For this review, take the finished solid that the model builds, in its own axes (mm). A direction names the side the tool comes from. Give positions to 0.01 mm unless a question says otherwise; leave off trailing zeros. Order: outer loops, then holes, each group sorted by start corner. A loop starts at its lowest first (then second) coordinate and runs counter-clockwise, first axis right, second up.
from build123d import *

# Parameters (mm, degrees)
SKETCH_1_W                   = 200
SKETCH_1_H                   = 80
EXTRUDE_1_DEPTH              = 10
SKETCH_3_R                   = 9
CUT_EXTRUDE_1_DEPTH          = 5
HOLE_WIZARD_M2_1_D           = 2.4
HOLE_WIZARD_M2_1_CBORE_D     = 5
HOLE_WIZARD_M2_1_CBORE_DEPTH = 7.7
SKETCH_13_R                  = 1.7
CUT_EXTRUDE_3_DEPTH          = 109.166538264
SKETCH_14_R                  = 3.25
CUT_EXTRUDE_4_DEPTH          = 109.166538264
FILLET1_R                    = 10
SKETCH3_W                    = 12
SKETCH3_H                    = 12
CUT_EXTRUDE2_DEPTH           = 109.166538264


with BuildPart() as part:
    # 草图1 → 凸台-拉伸1 (new body)
    with BuildSketch(Plane(origin=(0, 0, 0), x_dir=(1, 0, 0), z_dir=(0, 1, 0))):
        Rectangle(SKETCH_1_W, SKETCH_1_H)
    extrude(amount=EXTRUDE_1_DEPTH)

    # 草图3 → 切除-拉伸1 (cut)
    with BuildSketch(Plane(origin=(0, 10, 0), x_dir=(1, 0, 0), z_dir=(0, 1, 0))):
        with Locations(Location((-70, 0, 0), (0, 0, 270))):
            Circle(SKETCH_3_R)
    extrude(amount=-CUT_EXTRUDE_1_DEPTH, mode=Mode.SUBTRACT)

    # M2 六角凹头螺钉的柱形沉头孔1 (through all)
    with Locations(Plane(origin=(0, 0, 0), x_dir=(-1, 0, 0), z_dir=(0, -1, 0))):
        with Locations((47.5, 8), (77.5, 8), (77.5, -8), (47.5, -8)):
            CounterBoreHole(HOLE_WIZARD_M2_1_D / 2, HOLE_WIZARD_M2_1_CBORE_D / 2, HOLE_WIZARD_M2_1_CBORE_DEPTH)

    # 草图13 → 切除-拉伸3 (cut, through all)
    with BuildSketch(Plane(origin=(0, 10, 0), x_dir=(1, 0, 0), z_dir=(0, 1, 0))):
        with Locations(Location((-20, 31.5, 0), (0, 0, 270))):
            Circle(SKETCH_13_R)
        with Locations(Location((4, 31.5, 0), (0, 0, 270))):
            Circle(SKETCH_13_R)
        with Locations(Location((28, 31.5, 0), (0, 0, 270))):
            Circle(SKETCH_13_R)
        with Locations(Location((52, 31.5, 0), (0, 0, 270))):
            Circle(SKETCH_13_R)
        with Locations(Location((76, 31.5, 0), (0, 0, 270))):
            Circle(SKETCH_13_R)
        with Locations(Location((4, 10.5, 0), (0, 0, 270))):
            Circle(SKETCH_13_R)
        with Locations(Location((28, 10.5, 0), (0, 0, 270))):
            Circle(SKETCH_13_R)
        with Locations(Location((52, 10.5, 0), (0, 0, 270))):
            Circle(SKETCH_13_R)
        with Locations(Location((76, 10.5, 0), (0, 0, 270))):
            Circle(SKETCH_13_R)
        with Locations(Location((4, -10.5, 0), (0, 0, 270))):
            Circle(SKETCH_13_R)
        with Locations(Location((28, -10.5, 0), (0, 0, 270))):
            Circle(SKETCH_13_R)
        with Locations(Location((52, -10.5, 0), (0, 0, 270))):
            Circle(SKETCH_13_R)
        with Locations(Location((76, -10.5, 0), (0, 0, 270))):
            Circle(SKETCH_13_R)
        with Locations(Location((4, -31.5, 0), (0, 0, 270))):
            Circle(SKETCH_13_R)
        with Locations(Location((28, -31.5, 0), (0, 0, 270))):
            Circle(SKETCH_13_R)
        with Locations(Location((52, -31.5, 0), (0, 0, 270))):
            Circle(SKETCH_13_R)
        with Locations(Location((76, -31.5, 0), (0, 0, 270))):
            Circle(SKETCH_13_R)
        with Locations(Location((-20, 10.5, 0), (0, 0, 270))):
            Circle(SKETCH_13_R)
        with Locations(Location((-20, -10.5, 0), (0, 0, 270))):
            Circle(SKETCH_13_R)
        with Locations(Location((-20, -31.5, 0), (0, 0, 270))):
            Circle(SKETCH_13_R)
    extrude(amount=-CUT_EXTRUDE_3_DEPTH, mode=Mode.SUBTRACT)

    # 草图14 → 切除-拉伸4 (cut, through all)
    with BuildSketch(Plane(origin=(0, 10, 0), x_dir=(1, 0, 0), z_dir=(0, 1, 0))):
        with Locations(Location((-92.5, 32.5, 0), (0, 0, 270))):
            Circle(SKETCH_14_R)
        with Locations(Location((92.5, 32.5, 0), (0, 0, 90))):
            Circle(SKETCH_14_R)
        with Locations(Location((92.5, -32.5, 0), (0, 0, 270))):
            Circle(SKETCH_14_R)
        with Locations(Location((-92.5, -32.5, 0), (0, 0, 90))):
            Circle(SKETCH_14_R)
    extrude(amount=-CUT_EXTRUDE_4_DEPTH, mode=Mode.SUBTRACT)

    # Fillet1
    fillet1_edges = [part.edges().sort_by_distance(p)[0] for p in [
        (100, 5, 40),
        (-100, 5, 40),
        (-100, 5, -40),
        (100, 5, -40),
    ]]
    fillet(fillet1_edges, radius=FILLET1_R)

    # Sketch3 → Cut-Extrude2 (cut, through all)
    with BuildSketch(Plane(origin=(0, 10, 0), x_dir=(1, 0, 0), z_dir=(0, 1, 0))):
        with Locations((-62.5, -12)):
            Rectangle(SKETCH3_W, SKETCH3_H)
        with Locations((-62.5, 12)):
            Rectangle(SKETCH3_W, SKETCH3_H)
    extrude(amount=-CUT_EXTRUDE2_DEPTH, mode=Mode.SUBTRACT)


solid = part.part
1) We need section C-C on y = 2.75. Count the separate pieces of the cut face and the enclosed holes in it, then the cut area to 3 significant figures.
Answer sheet:
separate pieces: 1
enclosed holes: 30
area: 15,200 mm2
2) We need section A-A on z = 0. Give the boundary of the cut face in (x, y), then the cut area to 3 significant figures.
Answer sheet:
outline: (-100, 0) - (100, 0) - (100, 10) - (-61, 10) - (-61, 5) - (-79, 5) - (-79, 10) - (-100, 10) - close
area: 1,910 mm2
3) We need section B-B on x = -92.5. Give the boundary of the cut face in (y, z), then the cut area to 3 significant figures.
Answer sheet:
outline: (0, -39.68) - (10, -39.68) - (10, -35.75) - (0, -35.75) - close; (0, -29.25) - (10, -29.25) - (10, 29.25) - (0, 29.25) - close; (0, 35.75) - (10, 35.75) - (10, 39.68) - (0, 39.68) - close
area: 664 mm2
4) Draft analysis for pull direction Z (two halves, no side actions). For faces 1 (the face through (29.433, 5.07, -9.586)), 2 (the face through (96.99, 5.07, 37.15)), 3 (the face through (-100, 5, 0)), state which applies: +Z half, -Z half, draft (parallel to the pull), parting line (faces both ways), or undercut.
Answer sheet:
face 1: undercut
face 2: +Z half
face 3: draft
5) To check wall thickness, follow line 1 (Z direction, x = -47.5, y = 2.5); line 2 (Z direction, x = 76, y = 6.25); line 3 (Z direction, x = -47.5, y = 9.25). State the ranges of each line that lie inside material, in increasing order.
Answer sheet:
line 1: z = -40 to -10.5, -5.5 to 5.5, 10.5 to 40
line 2: z = -40 to -33.2, -29.8 to -12.2, -8.8 to 8.8, 12.2 to 29.8, 33.2 to 40
line 3: z = -40 to -9.2, -6.8 to 6.8, 9.2 to 40
6) Clearance check with a flat-ended pin moving along its axis: pin 1 (1.5 mm diameter, centred on x = -48.5, z = 7, fed in from -Y). State where the tip first meets the part, or that it passes through.
Answer sheet:
pin 1: stops at y = 7.7
7) Tool access review of faces 4 (the face through (-63, 5, 18)), 5 (the face through (-49, 7.7, -9)), 6 (the face through (-61, 8, 0)): name each direction out of +Z, -Z, +X, -X, +Y, -Y from which nothing blocks a thin tool from reaching the whole face with its end or side.
Answer sheet:
face 4: +Y, -Y
face 5: -Y
face 6: +Y
